from build123d import *

# Parameters (mm, degrees)
SKETCH_W        = 100
SKETCH_H        = 180
SKETCH_R        = 1.65
PAD_DEPTH       = 35
SKETCH001_R     = 3.3
SKETCH001_R_2   = 2.625
POCKET_DEPTH    = 35.001
SKETCH002_R     = 6
POCKET001_DEPTH = 25
SKETCH003_R     = 3
POCKET002_DEPTH = 25


with BuildPart() as part:
    # Sketch → Pad (new body)
    with BuildSketch(Plane.XZ):
        Rectangle(SKETCH_W, SKETCH_H)
        with Locations((10, 0)):
            Circle(SKETCH_R, mode=Mode.SUBTRACT)
        with Locations((-10, 0)):
            Circle(SKETCH_R, mode=Mode.SUBTRACT)
        with Locations((10, -80)):
            Circle(SKETCH_R, mode=Mode.SUBTRACT)
        with Locations((-10, -80)):
            Circle(SKETCH_R, mode=Mode.SUBTRACT)
    extrude(amount=PAD_DEPTH)

    # Sketch001 (on Face10 of Pad) → Pocket (cut, through all)
    with BuildSketch(Plane.XZ.offset(35)):
        with Locations((25, -80)):
            Circle(SKETCH001_R)
        with Locations((-25, -80)):
            Circle(SKETCH001_R)
        with Locations((25, 70)):
            Circle(SKETCH001_R)
        with Locations((-25, 70)):
            Circle(SKETCH001_R)
        with Locations((0, 82.5)):
            Circle(SKETCH001_R_2)
        with Locations((-37.5, -67.5)):
            Circle(SKETCH001_R_2)
        with Locations((37.5, -67.5)):
            Circle(SKETCH001_R_2)
    extrude(amount=-POCKET_DEPTH, mode=Mode.SUBTRACT)

    # Sketch002 (on Face5 of Pocket) → Pocket001 (cut)
    with BuildSketch(Plane.XZ.offset(35)):
        with Locations((25, 70)):
            Circle(SKETCH002_R)
        with Locations((-25, 70)):
            Circle(SKETCH002_R)
        with Locations((25, -80)):
            Circle(SKETCH002_R)
        with Locations((-25, -80)):
            Circle(SKETCH002_R)
        with Locations((-37.5, -67.5)):
            Circle(SKETCH002_R)
        with Locations((37.5, -67.5)):
            Circle(SKETCH002_R)
        with Locations((0, 82.5)):
            Circle(SKETCH002_R)
    extrude(amount=-POCKET001_DEPTH, mode=Mode.SUBTRACT)

    # Sketch003 (on Face4 of Pocket001) → Pocket002 (cut)
    with BuildSketch(Plane(origin=(0, 0, 0), x_dir=(1, 0, 0), z_dir=(0, 1, 0))):
        with Locations((-10, 80)):
            Circle(SKETCH003_R)
        with Locations((10, 80)):
            Circle(SKETCH003_R)
        with Locations((-10, 0)):
            Circle(SKETCH003_R)
        with Locations((10, 0)):
            Circle(SKETCH003_R)
    extrude(amount=-POCKET002_DEPTH, mode=Mode.SUBTRACT)


solid = part.part
Here's how the part is built. I have some questions about the finished solid (model axes, mm). A direction names the side the tool comes from. Coordinates: 2 decimals unless noted, no trailing zeros. Write each loop counter-clockwise with the first axis right and the second up, starting at its lowest first coordinate (ties: lowest second). Pieces come first, ordered by that corner, then holes.
1) If I drill on line 1 (X direction, y = -7.5, z = 69.5); line 2 (Z direction, x = 0, y = -22); line 3 (X direction, y = -17.5, z = -66), over which ranges is the centre line in solid material (lowest first)?
Filled in:
line 1: x = -50 to -28.26, -21.74 to 21.74, 28.26 to 50
line 2: z = -90 to 76.5, 88.5 to 90
line 3: x = -50 to -43.31, -31.69 to 31.69, 43.31 to 50
2) If we section it at D-D (x = 0): List the corners of the cut face in (y, z) for me (3 decimals).
Filled in:
outline: (-35, -90) - (0, -90) - (0, 79.875) - (-10, 79.875) - (-10, 76.5) - (-35, 76.5) - close; (-35, 88.5) - (-10, 88.5) - (-10, 85.125) - (0, 85.125) - (0, 90) - (-35, 90) - close
3) Thinking about a two-plate mould opening in Z: for faces 4 (the face through (20.58, -22.68, -75.94)), 5 (the face through (-1, 0, 1)), 6 (the face through (-1, -17, 90)), which applies, +Z half, -Z half, draft (parallel to the pull), parting line (faces both ways), or undercut?
Filled in:
face 4: undercut
face 5: draft
face 6: +Z half
4) Which directions (+Z, -Z, +X, -X, +Y, -Y) give clear straight access to the entire face, cutting with the end or side of a thin tool? Please do faces 1 (the face through (-12.4, -12.3, 1.8)), 2 (the face through (-8.476, -29.93, -0.632)), 3 (the face through (-35, -10, -69)).
Filled in:
face 1: +Y
face 2: +Y, -Y
face 3: -Y
5) If we section it at A-A (y = -21): Count the separate pieces of the cut face and the enclosed holes in it, plus the area to 3 significant figures.
Filled in:
separate pieces: 1
enclosed holes: 11
area: 17,100 mm2
6) If we section it at B-B (z = 82.5): List the corners of the cut face in (x, y) for me (3 decimals), plus the area to 3 significant figures.
Filled in:
outline: (-50, -35) - (-6, -35) - (-6, -10) - (-2.625, -10) - (-2.625, 0) - (-50, 0) - close; (2.625, -10) - (6, -10) - (6, -35) - (50, -35) - (50, 0) - (2.625, 0) - close
area: 3,150 mm2
7) I'm going to push flat-ended pins straight in: pin 1 (6 mm diameter, centred on x = 2.5, z = 83, fed in from -Y); pin 2 (3 mm diameter, centred on x = 11, z = 0, fed in from +Y). Where does each tip first touch, or does it pass through?
Filled in:
pin 1: stops at y = -10
pin 2: stops at y = -25
8) If we section it at C-C (x = 25): List the corners of the cut face in (y, z) for me.
Filled in:
outline: (-35, -90) - (0, -90) - (0, -83.3) - (-10, -83.3) - (-10, -86) - (-35, -86) - close; (-35, -74) - (-10, -74) - (-10, -76.7) - (0, -76.7) - (0, 66.7) - (-10, 66.7) - (-10, 64) - (-35, 64) - close; (-35, 76) - (-10, 76) - (-10, 73.3) - (0, 73.3) - (0, 90) - (-35, 90) - close
